Source: CAD feature listing. Evaluate the final solid. Frame: model axes, mm. A direction names the side the tool comes from. Coordinates: 2 decimals unless noted, no trailing zeros. Order: outer loops, then holes, each group sorted by start corner. A loop starts at its lowest first (then second) coordinate and runs counter-clockwise, first axis right, second up.
```python
from build123d import *

# Parameters (mm, degrees)
F1_DEPTH = 30
F2_R     = 10.259212
F3_DEPTH = 30


with BuildPart() as f1:
    # F0 (on Front) → F1 (new body)
    with BuildSketch(Plane.XZ):
        Polygon((29.64399, 25.039099), (-25.902519, 25.039099), (-25.902519, -26.765937), (29.64399, -26.765937), (47.775757, -26.765937), (47.775757, -11.224424), (29.64399, -11.224424), align=None)
    extrude(amount=F1_DEPTH)

    # F2 (on face) → F3 (cut)
    with BuildSketch(Plane(origin=(0, 0, 0), x_dir=(-1, 0, 0), z_dir=(0, 1, 0))):
        with Locations((-14.11511, 8.183153)):
            Circle(F2_R)
    extrude(amount=-F3_DEPTH, mode=Mode.SUBTRACT)


solid = f1.part
```
1. Access query for faces 1 (the face through (29.644, -15, 7)), 2 (the face through (2, -30, -1)). Directions: +Z, -Z, +X, -X, +Y, -Y. A direction counts if a zero-diameter tool reaches every point of the face in a straight line with its end or side. Return the directions, or none.
Findings:
face 1: +Z, +X, +Y, -Y
face 2: +Z, -Z, +X, -X, -Y
2. Section query C-C on y = -21. Return loops of the section in (x, z).
Findings:
outline: (-25.9, -26.77) - (47.78, -26.77) - (47.78, -11.22) - (29.64, -11.22) - (29.64, 25.04) - (-25.9, 25.04) - close; hole circle Ø20.52 at (14.12, 8.18)
3. Draft query along Z for faces 3 (the face through (2, -15, 25.039)), 4 (the face through (47.776, -15, -19)), 5 (the face through (22.256, -14.79, 1.941)), 6 (the face through (10, -15, -26.766)). Return one class per face: released by +Z, released by -Z, zero draft, split by the parting line, or undercut.
Findings:
face 3: released by +Z
face 4: zero draft
face 5: undercut
face 6: released by -Z
4. Ray query, line 1 (Z direction, x = 30.5, y = -23.5); line 2 (X direction, y = -24.5, z = 6); line 3 (Z direction, x = 23.5, y = -18.25). Return the intervals inside material, ascending.
Findings:
line 1: z = -26.77 to -11.22
line 2: x = -25.9 to 4.09, 24.14 to 29.64
line 3: z = -26.77 to 4.04, 12.33 to 25.04
5. Pin query (flat end, axial travel): P1, Ø14.5, axis at x = 37, y = -22, coming from the +Z side. Return the tip coordinate at first contact, or that it passes through.
Findings:
P1: stops at z = -11.22
6. Section query B-B on z = 17.5. Return loops of the section in (x, y).
Findings:
outline: (-25.9, -30) - (9.82, -30) - (9.82, 0) - (-25.9, 0) - close; (18.41, -30) - (29.64, -30) - (29.64, 0) - (18.41, 0) - close
7. Section query A-A on x = 21. Return loops of the section in (y, z).
Findings:
outline: (-30, -26.77) - (0, -26.77) - (0, 0.58) - (-30, 0.58) - close; (-30, 15.79) - (0, 15.79) - (0, 25.04) - (-30, 25.04) - close
8. Section query D-D on x = 32. Return loops of the section in (y, z), plus the area to 3 significant figures.
Findings:
outline: (-30, -26.77) - (0, -26.77) - (0, -11.22) - (-30, -11.22) - close
area: 466 mm2
